from build123d import *

# Parameters (mm, degrees)
F1_W     = 76.2
F1_H     = 76.2
F2_DEPTH = 228.6
F3_W     = 76.2
F3_H     = 76.2
F4_DEPTH = 76.2
F5_W     = 76.2
F5_H     = 76.2
F6_DEPTH = 76.2


# Not quite as in the source:
# - a variable given as a bare number and used for a length is read in inches; the dataset says mm whatever the document's units were


with BuildPart() as f2:
    # F1 (on Top) → F2 (new body)
    with BuildSketch(Plane.XY):
        Rectangle(F1_W, F1_H)
    extrude(amount=F2_DEPTH)

    # F3 (on face) → F4 (join)
    with BuildSketch(Plane.XZ.offset(38.1)):
        with Locations((0, 38.1)):
            Rectangle(F3_W, F3_H)
    extrude(amount=F4_DEPTH)

    # F5 (on face) → F6 (join)
    with BuildSketch(Plane(origin=(-38.1, 0, 0), x_dir=(0, -1, 0), z_dir=(-1, 0, 0))):
        with Locations((0, 114.3)):
            Rectangle(F5_W, F5_H)
    extrude(amount=F6_DEPTH)


solid = f2.part
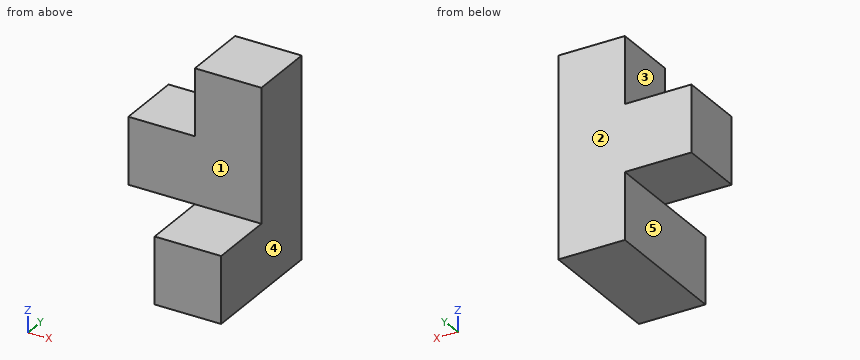
CAD build for the part. Positions are in the model's coordinates, mm. Face numbers are marked on the shaded views. A direction names the side the tool comes from. Give positions to 0.01 mm unless a question says otherwise; leave off trailing zeros. Write each loop counter-clockwise with the first axis right and the second up, starting at its lowest first coordinate (ties: lowest second). Pieces come first, ordered by that corner, then holes. Notation, with made-up numbers: (-12.75, 48.5) - (8.25, 48.5) arc R20 cw to (8.25, 72.5) - close; hole circle Ø4 at (-3.75, -2.75). An arc over 180 degrees is marked (long way). Put each result on its own line as item: value.
(1) Tool access for the marked faces 1, 2, 3, 4 and 5: list every direction of +Z, -Z, +X, -X, +Y, -Y with a clear straight run to the whole face (end or side of a thin tool).
Working result:
face 1: +Z, +X, -X, -Y
face 2: +Z, -Z, +X, -X, +Y
face 3: +Z, -X, +Y, -Y
face 4: +Z, -Z, +X, +Y, -Y
face 5: -Z, -X, +Y, -Y
(2) Saw through at D-D (x = -65). List the corners of the cut face in (y, z), then the cut area to 3 significant figures.
Working result:
outline: (-38.1, 76.2) - (38.1, 76.2) - (38.1, 152.4) - (-38.1, 152.4) - close
area: 5,810 mm^2
(3) Saw through at B-B (x = -30.5). List the corners of the cut face in (y, z), then the cut area to 3 significant figures.
Working result:
outline: (-114.3, 0) - (38.1, 0) - (38.1, 228.6) - (-38.1, 228.6) - (-38.1, 76.2) - (-114.3, 76.2) - close
area: 23,200 mm^2
(4) Saw through at C-C (z = 186). List the corners of the cut face in (x, y), then the cut area to 3 significant figures.
Working result:
outline: (-38.1, -38.1) - (38.1, -38.1) - (38.1, 38.1) - (-38.1, 38.1) - close
area: 5,810 mm^2
(5) Wall check: L1, parallel to Y at x = -62.5, z = 103; L2, parallel to Z at x = 26, y = -74. Give the ranges that are in metal, low to high.
Working result:
L1: -38.1 to 38.1
L2: 0 to 76.2
(6) Saw through at A-A (y = -23). List the corners of the cut face in (x, z), then the cut area to 3 significant figures.
Working result:
outline: (-114.3, 76.2) - (-38.1, 76.2) - (-38.1, 0) - (38.1, 0) - (38.1, 228.6) - (-38.1, 228.6) - (-38.1, 152.4) - (-114.3, 152.4) - close
area: 23,200 mm^2
(7) Drop flat-ended pins along their axis: pin 1 Ø23 at (x, y) = (-64.5, -13.5) entering from -Z; pin 2 Ø6 at (y, z) = (-69, 80.5) entering from +X; pin 3 Ø10 at (x, y) = (-26, -88) entering from +Z; pin 4 Ø23 at (x, y) = (-91.5, -10) entering from +Z. Give the stop position or say it passes through.
Working result:
pin 1: z = 76.2
pin 2: through
pin 3: z = 76.2
pin 4: z = 152.4
